```python
from build123d import *
from build123d.topology import SkipClean

# Parameters (mm, degrees)
CROQUIS1_R              = 1.7
SALIENTE_EXTRUIR1_DEPTH = 2
SALIENTE_EXTRUIR2_START = 10
CROQUIS2_R              = 1.7
SALIENTE_EXTRUIR2_DEPTH = 10
SALIENTE_EXTRUIR3_START = 8
CROQUIS3_R              = 1.7
SALIENTE_EXTRUIR3_DEPTH = 8
CROQUIS4_W              = 37.50862419
CROQUIS4_H              = 18.52759439
CORTAR_EXTRUIR1_DEPTH   = 10


with BuildPart() as part:
    # Croquis1 → Saliente-Extruir1 (new body)
    with BuildSketch(Plane.XY):
        with BuildLine():
            Line((77.885724234, 8.613797195), (71.814275766, 8.613797195))
            ThreePointArc((71.814275766, 8.613797195), (70.251539785, 10.455729214), (69.166367035, 12.613797195))
            ThreePointArc((69.166367035, 12.613797195), (65.166367035, 16.613797195), (61.166367035, 12.613797195))
            ThreePointArc((61.166367035, 12.613797195), (60.667946699, 10.638921667), (60.885724234, 8.613797195))
            Line((60.885724234, 8.613797195), (60.885724234, -9.113797195))
            ThreePointArc((60.885724234, -9.113797195), (60.667946699, -11.138921667), (61.166367035, -13.113797195))
            ThreePointArc((61.166367035, -13.113797195), (65.166367035, -17.113797195), (69.166367035, -13.113797195))
            ThreePointArc((69.166367035, -13.113797195), (70.251539785, -10.955729214), (71.814275766, -9.113797195))
            Line((71.814275766, -9.113797195), (77.885724234, -9.113797195))
            ThreePointArc((77.885724234, -9.113797195), (81.296227313, -10.565720048), (84.385724234, -12.613797195))
            ThreePointArc((84.385724234, -12.613797195), (87.885724234, -16.113797195), (91.385724234, -12.613797195))
            ThreePointArc((91.385724234, -12.613797195), (94.475221154, -10.565720048), (97.885724234, -9.113797195))
            Line((97.885724234, -9.113797195), (97.885724234, 8.613797195))
            ThreePointArc((97.885724234, 8.613797195), (94.475221154, 10.065720048), (91.385724234, 12.113797195))
            ThreePointArc((91.385724234, 12.113797195), (87.885724234, 15.613797195), (84.385724234, 12.113797195))
            ThreePointArc((84.385724234, 12.113797195), (81.296227313, 10.065720048), (77.885724234, 8.613797195))
        make_face()
        with Locations((65.166367035, -13.113797195)):
            Circle(CROQUIS1_R, mode=Mode.SUBTRACT)
        with Locations((65.166367035, 12.613797195)):
            Circle(CROQUIS1_R, mode=Mode.SUBTRACT)
        with Locations((87.885724234, 12.113797195)):
            Circle(CROQUIS1_R, mode=Mode.SUBTRACT)
        with Locations((87.885724234, -12.613797195)):
            Circle(CROQUIS1_R, mode=Mode.SUBTRACT)
    extrude(amount=SALIENTE_EXTRUIR1_DEPTH)

    # Croquis2 → Saliente-Extruir2 (add)
    # profile 1 of 4: a face of its own
    with SkipClean():  # the faces are left unmerged after this step: merging them gives an invalid solid
        with BuildSketch(Plane(origin=(0, 0, 0), x_dir=(-1, 0, 0), z_dir=(0, 0, -1)).offset(SALIENTE_EXTRUIR2_START)):
            with BuildLine():
                Line((-97.885724234, -9.113797195), (-77.885724234, -9.113797195))
                ThreePointArc((-77.885724234, -9.113797195), (-81.296227313, -10.565720048), (-84.385724234, -12.613797195))
                ThreePointArc((-84.385724234, -12.613797195), (-87.885724234, -16.113797195), (-91.385724234, -12.613797195))
                ThreePointArc((-91.385724234, -12.613797195), (-94.475221154, -10.565720048), (-97.885724234, -9.113797195))
            make_face()
            with Locations((-87.885724234, -12.613797195)):
                Circle(CROQUIS2_R, mode=Mode.SUBTRACT)
        # profile 2 of 4: a face of its own
        with BuildSketch(Plane(origin=(0, 0, 0), x_dir=(-1, 0, 0), z_dir=(0, 0, -1)).offset(SALIENTE_EXTRUIR2_START)):
            with BuildLine():
                Line((-97.885724234, 8.613797195), (-77.885724234, 8.613797195))
                ThreePointArc((-77.885724234, 8.613797195), (-81.296227313, 10.065720048), (-84.385724234, 12.113797195))
                ThreePointArc((-84.385724234, 12.113797195), (-87.885724234, 15.613797195), (-91.385724234, 12.113797195))
                ThreePointArc((-91.385724234, 12.113797195), (-94.475221154, 10.065720048), (-97.885724234, 8.613797195))
            make_face()
            with Locations((-87.885724234, 12.113797195)):
                Circle(CROQUIS2_R, mode=Mode.SUBTRACT)
        # profile 3 of 4: a face of its own
        with BuildSketch(Plane(origin=(0, 0, 0), x_dir=(-1, 0, 0), z_dir=(0, 0, -1)).offset(SALIENTE_EXTRUIR2_START)):
            with BuildLine():
                Line((-71.814275766, 8.613797195), (-60.885724234, 8.613797195))
                ThreePointArc((-60.885724234, 8.613797195), (-60.667946699, 10.638921667), (-61.166367035, 12.613797195))
                ThreePointArc((-61.166367035, 12.613797195), (-65.166367035, 16.613797195), (-69.166367035, 12.613797195))
                ThreePointArc((-69.166367035, 12.613797195), (-70.251539785, 10.455729214), (-71.814275766, 8.613797195))
            make_face()
            with Locations((-65.166367035, 12.613797195)):
                Circle(CROQUIS2_R, mode=Mode.SUBTRACT)
        # profile 4 of 4: a face of its own
        with BuildSketch(Plane(origin=(0, 0, 0), x_dir=(-1, 0, 0), z_dir=(0, 0, -1)).offset(SALIENTE_EXTRUIR2_START)):
            with BuildLine():
                Line((-71.814275766, -9.113797195), (-60.885724234, -9.113797195))
                ThreePointArc((-60.885724234, -9.113797195), (-60.667946699, -11.138921667), (-61.166367035, -13.113797195))
                ThreePointArc((-61.166367035, -13.113797195), (-65.166367035, -17.113797195), (-69.166367035, -13.113797195))
                ThreePointArc((-69.166367035, -13.113797195), (-70.251539785, -10.955729214), (-71.814275766, -9.113797195))
            make_face()
            with Locations((-65.166367035, -13.113797195)):
                Circle(CROQUIS2_R, mode=Mode.SUBTRACT)
        extrude(amount=-SALIENTE_EXTRUIR2_DEPTH)

    # Croquis3 → Saliente-Extruir3 (add)
    # profile 1 of 2: a face of its own
    with SkipClean():  # the faces are left unmerged after this step: merging them gives an invalid solid
        with BuildSketch(Plane(origin=(0, 0, -10), x_dir=(-1, 0, 0), z_dir=(0, 0, -1)).offset(SALIENTE_EXTRUIR3_START)):
            with BuildLine():
                Line((-71.814275766, 8.613797195), (-60.885724234, 8.613797195))
                ThreePointArc((-60.885724234, 8.613797195), (-60.667946699, 10.638921667), (-61.166367035, 12.613797195))
                ThreePointArc((-61.166367035, 12.613797195), (-65.166367035, 16.613797195), (-69.166367035, 12.613797195))
                ThreePointArc((-69.166367035, 12.613797195), (-70.251539785, 10.455729214), (-71.814275766, 8.613797195))
            make_face()
            with Locations((-65.166367035, 12.613797195)):
                Circle(CROQUIS3_R, mode=Mode.SUBTRACT)
        # profile 2 of 2: a face of its own
        with BuildSketch(Plane(origin=(0, 0, -10), x_dir=(-1, 0, 0), z_dir=(0, 0, -1)).offset(SALIENTE_EXTRUIR3_START)):
            with BuildLine():
                Line((-60.885724234, -9.113797195), (-71.814275766, -9.113797195))
                ThreePointArc((-71.814275766, -9.113797195), (-70.251539785, -10.955729214), (-69.166367035, -13.113797195))
                ThreePointArc((-69.166367035, -13.113797195), (-65.166367035, -17.113797195), (-61.166367035, -13.113797195))
                ThreePointArc((-61.166367035, -13.113797195), (-60.667946699, -11.138921667), (-60.885724234, -9.113797195))
            make_face()
            with Locations((-65.166367035, -13.113797195)):
                Circle(CROQUIS3_R, mode=Mode.SUBTRACT)
        extrude(amount=-SALIENTE_EXTRUIR3_DEPTH)

    # Croquis4 → Cortar-Extruir1 (cut)
    with SkipClean():  # the faces are left unmerged after this step: merging them gives an invalid solid
        with BuildSketch(Plane(origin=(0, 0, -10), x_dir=(-1, 0, 0), z_dir=(0, 0, -1))):
            with Locations((-79.131412139, -0.25)):
                Rectangle(CROQUIS4_W, CROQUIS4_H)
        extrude(amount=-CORTAR_EXTRUIR1_DEPTH, mode=Mode.SUBTRACT)


solid = part.part
```
Check sheet for the modelled part. Datum: model origin and axes. Units: mm. A direction names the side the tool comes from. Give positions to 0.01 mm unless a question says otherwise; leave off trailing zeros. Order: outer loops, then holes, each group sorted by start corner. A loop starts at its lowest first (then second) coordinate and runs counter-clockwise, first axis right, second up. Notation, with made-up numbers: (5, 47) -> (24, 47) arc R6 ccw to (24, 54) -> close; hole circle Ø5 at (26.25, -22.5). An arc over 180 degrees is marked (long way). Return JSON: item names as keys, results as strings.
1. Cross-section at B-B, the plane z = -13.75. Record the cut outline in (x, y), plus the area to 3 significant figures.
From the geometry:
{"outline": "(60.89, -9.11) arc R5.78 ccw to (61.17, -13.11) arc R4 ccw to (69.17, -13.11) arc R10.19 cw to (71.81, -9.11) -> close; (60.89, 8.61) -> (71.81, 8.61) arc R10.19 cw to (69.17, 12.61) arc R4 ccw to (61.17, 12.61) arc R5.78 ccw to start; hole circle Ø3.4 at (65.17, -13.11); hole circle Ø3.4 at (65.17, 12.61)", "area": "108 mm^2"}
2. Mould release check, pull along Z, two halves, no side actions. Record for faces 1 (the flat face through (97.886, 0, 1)), 2 (the flat face through (66.3, 10.9, -18)), 3 (the flat face through (66, 9.014, -5)), 4 (the flat face through (79, 0, 2)): +Z half, -Z half, draft (parallel to the pull), parting line (faces both ways), or undercut.
From the geometry:
{"face 1": "draft", "face 2": "-Z half", "face 3": "undercut", "face 4": "+Z half"}
3. Go/stop test with flat-tipped pins: P1, Ø4, axis at x = 65.17, y = -13.11, coming from the -Z side; P2, Ø8, axis at y = -2, z = -6.5, coming from the -X side; P3, Ø2, axis at x = 79, y = 4, coming from the -Z side; P4, Ø2, axis at x = 86, y = -11.5, coming from the -Z side. Record where each tip stops, or that it passes through.
From the geometry:
{"P1": "z = -18", "P2": "through", "P3": "z = 0", "P4": "z = -10"}
4. Set-up check for faces 5 (the flat face through (60.886, 0, 1)), 6 (the flat face through (66, 8.614, -14)), 7 (the flat face through (75, -9.114, 1)): record each of +Z, -Z, +X, -X, +Y, -Y from which the full face is reachable in a straight line by a thin tool's end or side.
From the geometry:
{"face 5": "+Z, -Z, -X", "face 6": "-Z, +X, -X", "face 7": "+Z, -Z, -Y"}
5. Cross-section at C-C, the plane x = 64.5. Record the cut outline in (y, z).
From the geometry:
{"outline": "(-17.06, -18) -> (-14.68, -18) -> (-14.68, 2) -> (-17.06, 2) -> close; (-11.55, -18) -> (-9.11, -18) -> (-9.11, -10) -> (-9.51, -10) -> (-9.51, 0) -> (9.01, 0) -> (9.01, -10) -> (8.61, -10) -> (8.61, -18) -> (11.05, -18) -> (11.05, 2) -> (-11.55, 2) -> close; (14.18, -18) -> (16.56, -18) -> (16.56, 2) -> (14.18, 2) -> close"}
6. Material ranges on probe 1 along X at (y, z) = (-14, -8.75); probe 2 along Y at (x, z) = (87.5, -2.75); probe 3 along Z at (x, y) = (69.5, -8.5), recorded low to high. Write a range as [from, to].
From the geometry:
{"probe 1": "[61.27, 63.72], [66.62, 69.07], [84.67, 86.9], [88.87, 91.1]", "probe 2": "[-16.09, -14.27], [-10.96, -9.51], [9.01, 10.46], [13.77, 15.59]", "probe 3": "[0, 2]"}
7. Cross-section at D-D, the plane x = 68.5. Record the cut outline in (y, z), plus the area to 3 significant figures.
From the geometry:
{"outline": "(-15.32, -18) -> (-9.11, -18) -> (-9.11, -10) -> (-9.51, -10) -> (-9.51, 0) -> (9.01, 0) -> (9.01, -10) -> (8.61, -10) -> (8.61, -18) -> (14.82, -18) -> (14.82, 2) -> (-15.32, 2) -> close", "area": "276 mm^2"}
8. Cross-section at A-A, the plane z = -0.5. Record the cut outline in (x, y), plus the area to 3 significant figures.
From the geometry:
{"outline": "(60.78, -9.51) arc R5.78 ccw to (61.17, -13.11) arc R4 ccw to (69.17, -13.11) arc R10.19 cw to (71.41, -9.51) -> close; (60.78, 9.01) -> (71.41, 9.01) arc R10.19 cw to (69.17, 12.61) arc R4 ccw to (61.17, 12.61) arc R5.78 ccw to start; (79.01, -9.51) arc R20.29 cw to (84.39, -12.61) arc R3.5 ccw to (91.39, -12.61) arc R20.29 cw to (96.76, -9.51) -> close; (79.01, 9.01) -> (96.76, 9.01) arc R20.29 cw to (91.39, 12.11) arc R3.5 ccw to (84.39, 12.11) arc R20.29 cw to start; hole circle Ø3.4 at (65.17, -13.11); hole circle Ø3.4 at (65.17, 12.61); hole circle Ø3.4 at (87.89, -12.61); hole circle Ø3.4 at (87.89, 12.11)", "area": "192 mm^2"}
